from build123d import *

# Parameters (mm, degrees)
SKETCH1_R                  = 5
BOSS_EXTRUDE1_DEPTH        = 198
OTW_R_GWINTOWANY_M52_D     = 4.2
OTW_R_GWINTOWANY_M52_DEPTH = 20
OTW_R_GWINTOWANY_M52_TIP   = 1.2618073
SZKIC7_R                   = 5.5
SZKIC7_R_2                 = 4
WYTNIJ_WYCI_GNI_CIE1_DEPTH = 10


with BuildPart() as part:
    # Sketch1 → Boss-Extrude1 (new body)
    with BuildSketch(Plane.XY):
        Circle(SKETCH1_R)
    extrude(amount=BOSS_EXTRUDE1_DEPTH)

    # Otwór gwintowany M52
    with Locations(Plane(origin=(0, 0, 0), x_dir=(-1, 0, 0), z_dir=(0, 0, -1))):
        with Locations((0, 0)):
            Hole(OTW_R_GWINTOWANY_M52_D / 2, depth=OTW_R_GWINTOWANY_M52_DEPTH)
            with Locations((0, 0, -(OTW_R_GWINTOWANY_M52_DEPTH + OTW_R_GWINTOWANY_M52_TIP / 2))):  # 118° drill point
                Cone(0, OTW_R_GWINTOWANY_M52_D / 2, OTW_R_GWINTOWANY_M52_TIP, mode=Mode.SUBTRACT)

    # Szkic7 → Wytnij-wyciągnięcie1 (cut)
    with BuildSketch(Plane.XY.offset(198)):
        Circle(SZKIC7_R)
        Circle(SZKIC7_R_2, mode=Mode.SUBTRACT)
    extrude(amount=-WYTNIJ_WYCI_GNI_CIE1_DEPTH, mode=Mode.SUBTRACT)


solid = part.part
Geometry: final body of the model. Coordinates: model frame, mm. Coordinates: 2 decimals unless noted, no trailing zeros. Order: outer loops, then holes, each group sorted by start corner. A loop starts at its lowest first (then second) coordinate and runs counter-clockwise, first axis right, second up.
(1) First-contact query: pin 1 (5 mm diameter, centred on y = -4, z = 33.5, fed in from +X); pin 2 (2 mm diameter, centred on x = -2, z = 106.5, fed in from +Y). Flat tips, straight axial feed; report the tip coordinate or a pass-through.
(2) Material intervals for probe 1 along X at (y, z) = (0, 5); probe 2 along X at (y, z) = (0.25, 102), sorted ascending.
(3) Section query A-A (z = 46.5). Return the cut outline in (x, y).
(4) Draft query along X for faces 1 (the face through (-0.867, -3.905, 193.07)), 2 (the face through (2.003, 0.631, 10.14)), 3 (the face through (1, -2.2, 0)). Return one class per face: pulls with the +X half, pulls with the -X half, needs draft (parallel to the pull), parting line crosses it, or undercut.
Solution:
1. pin 1: stops at x = 4.77
1. pin 2: stops at y = 4.9
2. probe 1: x = -5 to -2.1, 2.1 to 5
2. probe 2: x = -4.99 to 4.99
3. outline: circle Ø10 at (0, 0)
4. face 1: parting line crosses it
4. face 2: undercut
4. face 3: needs draft
